Print and shaded views of the part. All mm, measured from the part's lowest x, y and z. A direction names the side the tool comes from. Give positions to 0.01 mm unless a question says otherwise; leave off trailing zeros. Write each loop counter-clockwise with the first axis right and the second up, starting at its lowest first coordinate (ties: lowest second). Pieces come first, ordered by that corner, then holes. Notation, with made-up numbers: M 17,5 L 39,5 A35 cw 39,37 Z; hole C 1.5,24.25 d8. An arc over 180 degrees is marked long. One line per question, with ' | ' between items. Start each with the question number.
1. Cut at A-A, the plane y = 7.45. Write the cut outline in (x, z).
2. Wall check: L1, parallel to Z at x = 12.5, y = 6; L2, parallel to X at y = 7.5, z = 1.5; L3, parallel to Z at x = 1.5, y = 6. Give the ranges that are in metal, low to high.
3. Cut at B-B, the plane x = 7.45. Write the cut outline in (y, z), then the cut area to 3 significant figures.
4. Cut at C-C, the plane z = 6.25. Write the cut outline in (x, y).
5. Cut at D-D, the plane y = 3. Write the cut outline in (x, z), then the cut area to 3 significant figures.
6. Which spindle directions (+Z, -Z, +X, -X, +Y, -Y) get a long thin tool onto all of the face, cutting with end or side? Do the marked faces 1 and 2. Say none if no direction does.
7. Flat gauge pins, fed straight in: pin 1 (5 mm diameter, centred on y = 11.5, z = 4.5, fed in from +X); pin 2 (3 mm diameter, centred on x = 2, z = 5.5, fed in from +Y); pin 3 (4 mm diameter, centred on y = 4.5, z = 7.5, fed in from -X); pin 4 (1 mm diameter, centred on y = 1.5, z = 1, fed in from -X). Where does each tip first touch, or does it go through?
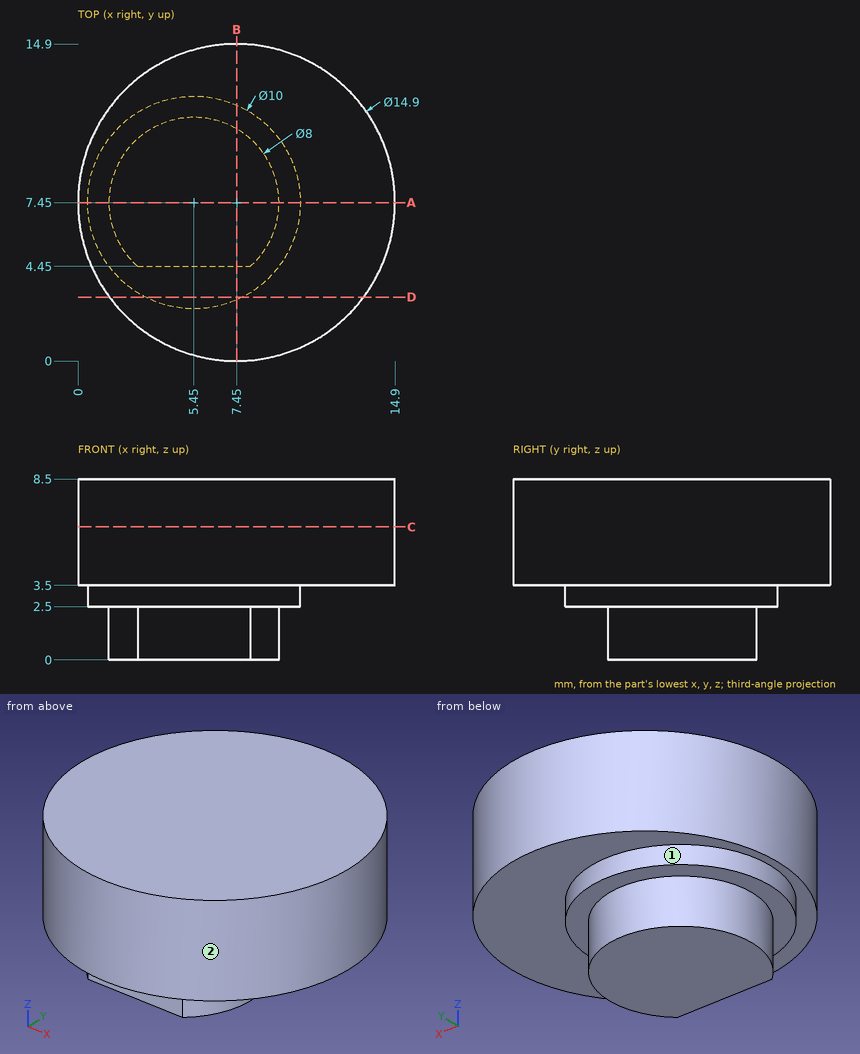
Here are the results:
1) outline: M 0,3.5 L 0.45,3.5 L 0.45,2.5 L 1.45,2.5 L 1.45,0 L 9.45,0 L 9.45,2.5 L 10.45,2.5 L 10.45,3.5 L 14.9,3.5 L 14.9,8.5 L 0,8.5 Z
2) L1: 3.5 to 8.5 | L2: 1.45 to 9.45 | L3: 2.5 to 8.5
3) outline: M 0,3.5 L 2.87,3.5 L 2.87,2.5 L 4.45,2.5 L 4.45,0 L 10.91,0 L 10.91,2.5 L 12.03,2.5 L 12.03,3.5 L 14.9,3.5 L 14.9,8.5 L 0,8.5 Z | area: 99.8 mm^2
4) outline: C 7.45,7.45 d14.9
5) outline: M 1.48,3.5 L 3.17,3.5 L 3.17,2.5 L 7.73,2.5 L 7.73,3.5 L 13.42,3.5 L 13.42,8.5 L 1.48,8.5 Z | area: 64.3 mm^2
6) face 1: -Z | face 2: +Z, -Z
7) pin 1: x = 14.74 | pin 2: y = 13.77 | pin 3: x = 0.06 | pin 4: through
